Study the drawing (mm; zero at the part's minimum x, y, z) and answer. Round coordinates to 2 decimals unless told otherwise and drop trailing zeros. Write each loop counter-clockwise with the first axis right and the second up, starting at its lowest first coordinate (ties: lowest second). Pieces come first, ordered by that corner, then holes.
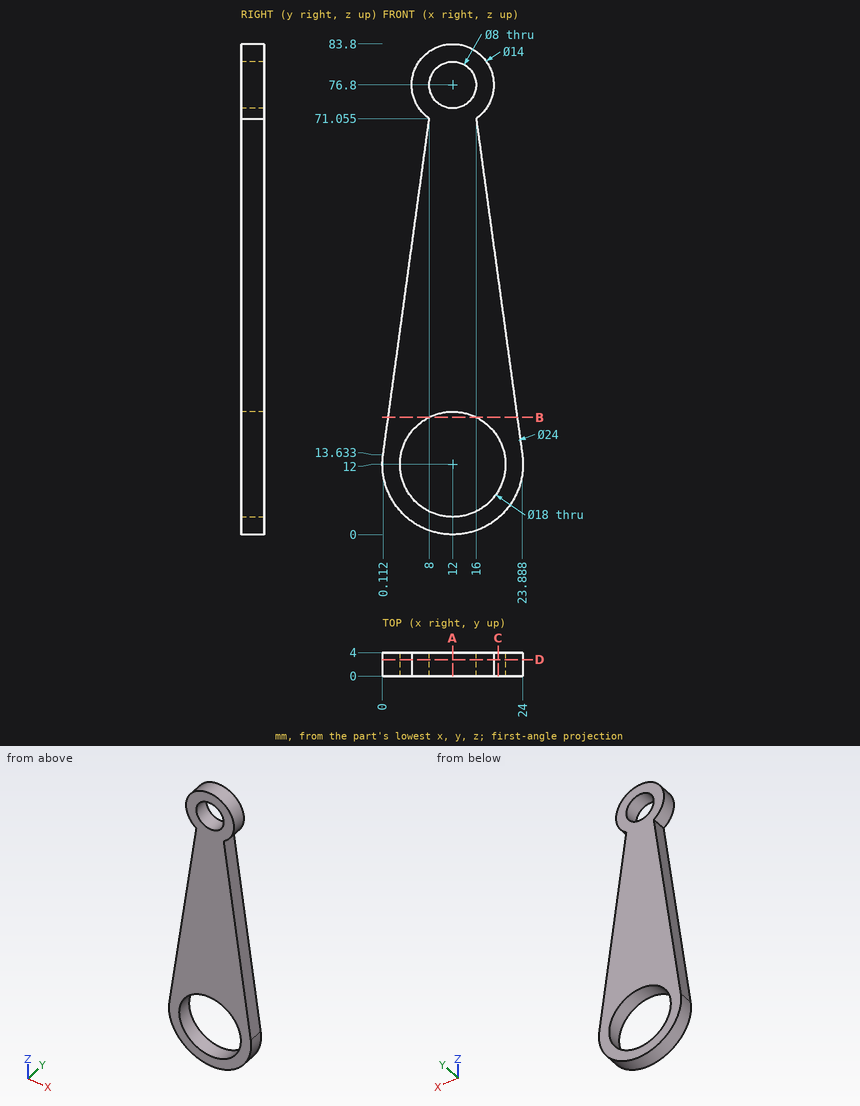
1. Section D-D on y = 2.8 is taken. Determine the outline of the cut face in (x, z) (1 decimal).
Geometry says:
outline: (0.1, 13.6) arc R12 ccw (long way) to (23.9, 13.6) - (16, 71.1) arc R7 ccw (long way) to (8, 71.1) - close; hole circle Ø18 at (12, 12); hole circle Ø8 at (12, 76.8)
2. Straight lines are drawn through the part: line 1 along Z through (x, y) = (12.75, 3.35); line 2 along Z through (x, y) = (13.5, 0.2) (1 decimal); line 3 along X through (y, z) = (0.9, 76) (1 decimal). For each, find the intervals that lie inside material, in ascending order.
Geometry says:
line 1: z = 0.02 to 3.03, 20.97 to 72.87, 80.73 to 83.76
line 2: z = 0.1 to 3.1, 20.9 to 73.1, 80.5 to 83.6
line 3: x = 5 to 8.1, 15.9 to 19
3. Section A-A on x = 12 is taken. Determine the outline of the cut face in (y, z), plus the area to 3 significant figures.
Geometry says:
outline: (0, 0) - (4, 0) - (4, 3) - (0, 3) - close; (0, 21) - (4, 21) - (4, 72.8) - (0, 72.8) - close; (0, 80.8) - (4, 80.8) - (4, 83.8) - (0, 83.8) - close
area: 231 mm2
4. Section B-B on z = 20 is taken. Determine the outline of the cut face in (x, y).
Geometry says:
outline: (0.99, 0) - (7.88, 0) - (7.88, 4) - (0.99, 4) - close; (16.12, 0) - (23.01, 0) - (23.01, 4) - (16.12, 4) - close
5. Given pin 1 (1.5 mm diameter, centred on y = 3.5, z = 75.5, fed in from +X), flat-ended and moving along its own axis, determine where the tip first touches the part or whether it passes through.
Geometry says:
pin 1: stops at x = 18.98
6. Section C-C on x = 19.75 is taken. Determine the outline of the cut face in (y, z) (1 decimal).
Geometry says:
outline: (0, 2.8) - (4, 2.8) - (4, 7.4) - (0, 7.4) - close; (0, 16.6) - (4, 16.6) - (4, 43.8) - (0, 43.8) - close
